Model file for the job. Use its own axes, mm. Face numbers are marked on the shaded views. A direction names the side the tool comes from. Coordinates: 2 decimals unless noted, no trailing zeros. Write each loop counter-clockwise with the first axis right and the second up, starting at its lowest first coordinate (ties: lowest second). Pieces come first, ordered by that corner, then holes. Notation, with made-up numbers: M 16.25,1 L 60.25,1 A25 ccw 60.25,39 Z; hole C -26,19 d5. An arc over 180 degrees is marked long. Put each result on its own line as item: value. Start each with the question number.
Q1. Drill centre lines: line 1 along X through (y, z) = (-10, 40); line 2 along X through (y, z) = (-19, -87); line 3 along Z through (x, y) = (10.5, -26.5) (3 decimals). Where is each one in solid material? Low to high.
Q2. Cut at A-A (z = 51.5). Write the cut outline in (x, y).
Q3. Cut at C-C (z = 4). Write the cut outline in (x, y), then the cut area to 3 significant figures.
Q4. Which spindle directions (+Z, -Z, +X, -X, +Y, -Y) get a long thin tool onto all of the face, cutting with end or side? Do the marked faces 1, 2 and 3. Say none if no direction does.
Q5. Drop flat-ended pins along their axis: pin 1 (15.5 mm diameter, centred on x = 10.5, y = -11.5, fed in from +Z); pin 2 (12 mm diameter, centred on x = 35.5, z = 17.5, fed in from -Y); pin 3 (10.5 mm diameter, centred on y = -5.5, z = 101, fed in from -X). Give the stop position or say it passes through.
Q6. Pull direction X, two halves, no side cores. Call the marked faces 4, 5 and 6: pulls with the +X half, pulls with the -X half, needs draft (parallel to the pull), parting line crosses it, or undercut.
Q7. Cut at D-D (z = -21). Write the cut outline in (x, y).
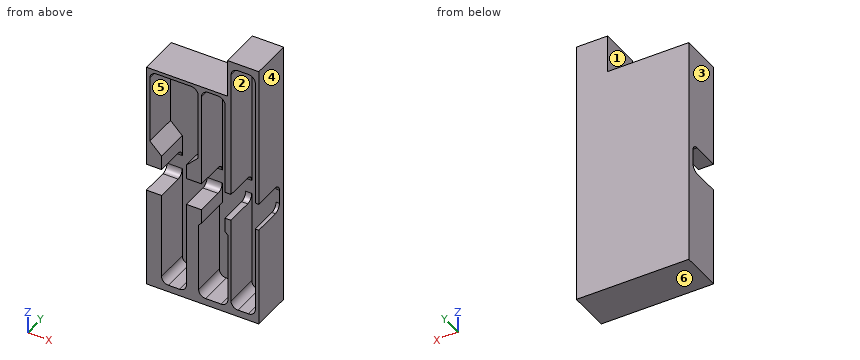
```python
from build123d import *

# Parameters (mm, degrees)
F0_W          = 103.505
F0_H          = 247.65
F1_DEPTH      = 31.75
F1_DEPTH_BACK = 6.35
F2_W          = 22.352
F2_H          = 234.95
F3_DEPTH      = 31.75
F4_R          = 6.35
F5_W          = 74.803
F5_H          = 34.925
F6_DEPTH      = 38.101
F7_W          = 103.505
F7_H          = 25.4
F8_DEPTH      = 31.75
F9_R          = 6.35


with BuildPart() as f1:
    # F0 (on Front) → F1 (new body, two sides)
    with BuildSketch(Plane.XZ) as f1_sk:
        Rectangle(F0_W, F0_H)
    extrude(amount=F1_DEPTH)
    extrude(f1_sk.sketch, amount=-F1_DEPTH_BACK)

    # F2 (on Front) → F3 (cut, through all)
    with BuildSketch(Plane.XZ):
        with Locations((37.4015, 0)):
            Rectangle(F2_W, F2_H)
        Polygon((20.6375, 85.725), (-0.9525, 85.725), (-0.9525, -44.958), (-3.6195, -47.625), (-3.6195, -117.475), (23.3045, -117.475), (23.3045, -47.625), (20.6375, -44.958), align=None)
        Polygon((-37.7825, 6.858), (-37.7825, -117.475), (-14.9225, -117.475), (-14.9225, 6.858), (-4.1275, 17.653), (-4.1275, 85.725), (-48.5775, 85.725), (-48.5775, 17.653), align=None)
    extrude(amount=F3_DEPTH, mode=Mode.SUBTRACT)

    # F4
    f4_edges = [f1.edges().sort_by_distance(p)[0] for p in [
        (-48.5775, -15.875, 85.725),
        (-4.1275, -15.875, 85.725),
        (20.6375, -15.875, 85.725),
        (-0.9525, -15.875, 85.725),
        (-14.9225, -15.875, -117.475),
        (-37.7825, -15.875, -117.475),
        (23.3045, -15.875, -117.475),
        (-3.6195, -15.875, -117.475),
        (48.5775, -15.875, 117.475),
        (26.2255, -15.875, 117.475),
        (26.2255, -15.875, -117.475),
        (48.5775, -15.875, -117.475),
    ]]
    fillet(f4_edges, radius=F4_R)

    # F5 (on face) → F6 (cut, through all)
    with BuildSketch(Plane.XZ.offset(31.75)):
        with Locations((-14.351, 106.3625)):
            Rectangle(F5_W, F5_H)
    extrude(amount=-F6_DEPTH, mode=Mode.SUBTRACT)

    # F7 (on face) → F8 (cut)
    with BuildSketch(Plane.XZ.offset(31.75)):
        with Locations((0, -19.05)):
            Rectangle(F7_W, F7_H)
    extrude(amount=-F8_DEPTH, mode=Mode.SUBTRACT)

    # F9
    f9_edges = [f1.edges().sort_by_distance(p)[0] for p in [
        (-44.7675, 0, -6.35),
        (50.165, 0, -6.35),
        (23.4315, 0, -6.35),
        (-7.9375, 0, -6.35),
        (-44.7675, 0, -31.75),
        (-7.9375, 0, -31.75),
        (23.4315, 0, -31.75),
        (50.165, 0, -31.75),
    ]]
    fillet(f9_edges, radius=F9_R)


solid = f1.part
```
Computed values:
1. line 1: -51.75 to -48.58, -4.13 to -0.95, 20.64 to 26.23, 48.58 to 51.75
1. line 2: -51.75 to -37.78, -14.92 to -3.62, 23.3 to 26.23, 48.58 to 51.75
1. line 3: -123.825 to -117.475, 85.725 to 88.9
2. outline: M -51.75,-31.75 L -48.58,-31.75 L -48.58,0 L -4.13,0 L -4.13,-31.75 L -0.95,-31.75 L -0.95,0 L 20.64,0 L 20.64,-31.75 L 26.23,-31.75 L 26.23,0 L 48.58,0 L 48.58,-31.75 L 51.75,-31.75 L 51.75,6.35 L -51.75,6.35 Z
3. outline: M -51.75,-31.75 L -37.78,-31.75 L -37.78,0 L -14.92,0 L -14.92,-31.75 L -0.95,-31.75 L -0.95,0 L 20.64,0 L 20.64,-31.75 L 26.23,-31.75 L 26.23,0 L 48.58,0 L 48.58,-31.75 L 51.75,-31.75 L 51.75,6.35 L -51.75,6.35 Z
3. area: 1,820 mm2
4. face 1: +Z, -X, +Y, -Y
4. face 2: -Y
4. face 3: +Z, -Z, -X, +Y, -Y
5. pin 1: z = 88.9
5. pin 2: y = 0
5. pin 3: x = 23.05
6. face 4: pulls with the +X half
6. face 5: undercut
6. face 6: needs draft
7. outline: M -51.75,0 L 51.75,0 L 51.75,6.35 L -51.75,6.35 Z
